Source: CAD feature listing. Evaluate the final solid. Frame: model axes, mm. Face numbers are marked on the shaded views. A direction names the side the tool comes from. Give positions to 0.01 mm unless a question says otherwise; leave off trailing zeros. Order: outer loops, then holes, each group sorted by start corner. A loop starts at its lowest first (then second) coordinate and runs counter-clockwise, first axis right, second up. Notation, with made-up numbers: (-24.5, 38) -> (-16.5, 38) arc R26 cw to (-16.5, 67) -> close; hole circle Ø1 at (-33, 39.5). An arc over 180 degrees is marked (long way). Use CSV: the item, a comma, the result in double quotes.
```python
from build123d import *

# Parameters (mm, degrees)
SKETCH_1_R               = 50
EXTRUDE_1_DEPTH          = 15
SKETCH_2_R               = 19
EXTRUDE_2_DEPTH          = 2.5
CUT_EXTRUDE_1_DEPTH      = 73.284161474
CUT_EXTRUDE_1_DEPTH_BACK = 73.284161474
SKETCH_3_R               = 5.5


with BuildPart() as part:
    # 草图1 → 凸台-拉伸1 (new body)
    with BuildSketch(Plane(origin=(0, 0, 0), x_dir=(1, 0, 0), z_dir=(0, 1, 0))):
        with Locations(Location((0, 0, 0), (0, 0, 270))):
            Circle(SKETCH_1_R)
    extrude(amount=EXTRUDE_1_DEPTH)

    # 草图2 → 凸台-拉伸2 (add)
    with BuildSketch(Plane(origin=(0, 15, 0), x_dir=(1, 0, 0), z_dir=(0, 1, 0))):
        with Locations(Location((0, 0, 0), (0, 0, 270))):
            Circle(SKETCH_2_R)
    extrude(amount=EXTRUDE_2_DEPTH)

    # 草图3 → 切除-拉伸1 (cut, two sides: drawn at the far end of the back side and taken through both)
    with BuildSketch(Plane(origin=(0, 15, 0), x_dir=(1, 0, 0), z_dir=(0, 1, 0)).offset(-CUT_EXTRUDE_1_DEPTH_BACK)):
        with Locations(Location((26.162950904, 26.162950904, 0), (0, 0, 270))):
            Circle(SKETCH_3_R)
        with Locations(Location((26.162950904, -26.162950904, 0), (0, 0, 270))):
            Circle(SKETCH_3_R)
        with Locations(Location((-26.162950904, -26.162950904, 0), (0, 0, 270))):
            Circle(SKETCH_3_R)
        with Locations(Location((-26.162950904, 26.162950904, 0), (0, 0, 270))):
            Circle(SKETCH_3_R)
    extrude(amount=CUT_EXTRUDE_1_DEPTH + CUT_EXTRUDE_1_DEPTH_BACK, mode=Mode.SUBTRACT)


solid = part.part
```
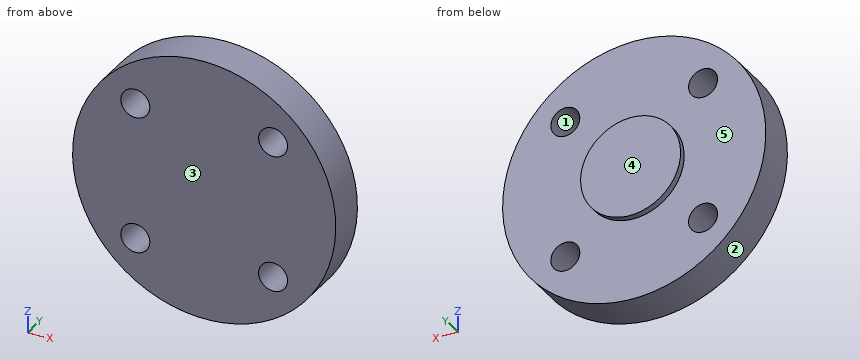
1. Section query A-A on z = 30.5. Return loops of the section in (x, y), plus the area to 3 significant figures.
Answer below:
outline,"(-39.62, 0) -> (-29.55, 0) -> (-29.55, 15) -> (-39.62, 15) -> close; (-22.78, 0) -> (22.78, 0) -> (22.78, 15) -> (-22.78, 15) -> close; (29.55, 0) -> (39.62, 0) -> (39.62, 15) -> (29.55, 15) -> close"
area,"986 mm²"
2. Section query D-D on z = 0. Return loops of the section in (x, y).
Answer below:
outline,"(-50, 0) -> (50, 0) -> (50, 15) -> (19, 15) -> (19, 17.5) -> (-19, 17.5) -> (-19, 15) -> (-50, 15) -> close"
3. Mould query, pull axis Z, two halves, no side actions, for the marked faces 1, 2 and 3. Classes: released by +Z, released by -Z, zero draft, split by the parting line, or undercut.
Answer below:
face 1,"undercut"
face 2,"split by the parting line"
face 3,"zero draft"
4. Section query B-B on x = 0. Return loops of the section in (y, z), plus the area to 4 significant figures.
Answer below:
outline,"(0, -50) -> (15, -50) -> (15, -19) -> (17.5, -19) -> (17.5, 19) -> (15, 19) -> (15, 50) -> (0, 50) -> close"
area,"1,595 mm²"
5. Ray query, line 1 along X through (y, z) = (5.75, -27); line 2 along X through (y, z) = (1, 26.5); line 3 along Z through (x, y) = (25, 5). Return the intervals inside material, ascending.
Answer below:
line 1,"x = -42.08 to -31.6, -20.73 to 20.73, 31.6 to 42.08"
line 2,"x = -42.4 to -31.65, -20.67 to 20.67, 31.65 to 42.4"
line 3,"z = -43.3 to -31.54, -20.79 to 20.79, 31.54 to 43.3"
6. Pin query (flat end, axial travel): P1, Ø12.5, axis at x = -26.16, z = -26.16, coming from the +Y side; P2, Ø1, axis at y = 7, z = -27.5, coming from the +X side; P3, Ø1, axis at x = 33.5, y = 9, coming from the -Z side. Return the tip coordinate at first contact, or that it passes through.
Answer below:
P1,"stops at y = 15"
P2,"stops at x = 42.08"
P3,"stops at z = -37.56"
7. Access query for the marked faces 4 and 5. Directions: +Z, -Z, +X, -X, +Y, -Y. A direction counts if a zero-diameter tool reaches every point of the face in a straight line with its end or side. Return the directions, or none.
Answer below:
face 4,"+Z, -Z, +X, -X, +Y"
face 5,"+Y"
8. Section query C-C on y = 12.5. Return loops of the section in (x, z), plus the area to 3 significant figures.
Answer below:
outline,"circle Ø100 at (0, 0); hole circle Ø11 at (-26.16, -26.16); hole circle Ø11 at (-26.16, 26.16); hole circle Ø11 at (26.16, -26.16); hole circle Ø11 at (26.16, 26.16)"
area,"7,470 mm²"
